Can you work these out from the model? Positions are in its coordinate system, mm. Face numbers are marked on the shaded views. A direction names the side the tool comes from. Round coordinates to 2 decimals unless told otherwise and drop trailing zeros. Write each loop counter-clockwise with the first axis right and the second up, starting at its lowest first coordinate (ties: lowest second). Pieces come first, ordered by that corner, then holes.
Q1. If we section it at C-C (x = 11): Please give me the cut outline in (y, z), plus the area to 3 significant figures.
Q2. For the marked faces 1, 2 and 3, which set-ups out of +Z, -Z, +X, -X, +Y, -Y let a thin tool reach every point of the face, with its end or its side?
Q3. If we section it at D-D (y = 6): Please give me the cut outline in (x, z), plus the area to 3 significant figures.
Q4. If we section it at B-B (z = 2.25): Please give me the cut outline in (x, y), plus the area to 3 significant figures.
Q5. I'm going to push flat-ended pins straight in: pin 1 Ø1.5 at (y, z) = (-16, 2) entering from +X; pin 2 Ø4.5 at (x, y) = (11.71, -15.62) entering from +Z; pin 3 Ø0.7 at (y, z) = (-16, 1.5) entering from -X. Where does each tip first touch, or does it pass through?
Q6. If we section it at A-A (x = 5.5): Please give me the cut outline in (y, z).
Q7. Please list where these lines run through material, in increasing order: line 1 along Y through (x, z) = (-5, 2); line 2 along X through (y, z) = (0, 2.25); line 3 along Y through (x, z) = (-6, 6.25).
from build123d import *

# Parameters (mm, degrees)
SKETCH1_R           = 16.5
SKETCH1_R_2         = 2.4
SKETCH1_R_3         = 1.4
BOSS_EXTRUDE1_DEPTH = 3
BOSS_EXTRUDE2_START = -3
SKETCH3_R           = 1.4
BOSS_EXTRUDE2_DEPTH = 3
SKETCH4_W           = 33
SKETCH4_H           = 12
SKETCH4_R           = 1.4
BOSS_EXTRUDE3_DEPTH = 5.5
SKETCH5_W           = 33
SKETCH5_H           = 9
CUT_EXTRUDE1_DEPTH  = 6.5
FILLET1_R           = 3
CHAMFER1_SIZE       = 1


with BuildPart() as part:
    # Sketch1 → Boss-Extrude1 (new body)
    # profile 1 of 5: a face of its own
    with BuildSketch(Plane.XY):
        with Locations((3.7111495, -7.618539739)):
            Circle(SKETCH1_R)
        with BuildLine():
            ThreePointArc((-4.2888505, -2.018539739), (-5.985906775, 2.078516536), (-1.8888505, 0.381460261))
            Line((-1.8888505, 0.381460261), (-1.8888505, 1.781460261))
            Line((-1.8888505, 1.781460261), (9.3111495, 1.781460261))
            Line((9.3111495, 1.781460261), (9.3111495, 0.381460261))
            ThreePointArc((9.3111495, 0.381460261), (11.7111495, 2.781460261), (14.1111495, 0.381460261))
            ThreePointArc((14.1111495, 0.381460261), (13.408205775, -1.315596014), (11.7111495, -2.018539739))
            Line((11.7111495, -2.018539739), (13.1111495, -2.018539739))
            Line((13.1111495, -2.018539739), (13.1111495, -13.218539739))
            Line((13.1111495, -13.218539739), (11.7111495, -13.218539739))
            ThreePointArc((11.7111495, -13.218539739), (13.408205775, -13.921483464), (14.1111495, -15.618539739))
            ThreePointArc((14.1111495, -15.618539739), (11.7111495, -18.018539739), (9.3111495, -15.618539739))
            Line((9.3111495, -15.618539739), (9.3111495, -17.018539739))
            Line((9.3111495, -17.018539739), (-1.8888505, -17.018539739))
            Line((-1.8888505, -17.018539739), (-1.8888505, -15.618539739))
            ThreePointArc((-1.8888505, -15.618539739), (-5.985906775, -17.315596014), (-4.2888505, -13.218539739))
            Line((-4.2888505, -13.218539739), (-5.6888505, -13.218539739))
            Line((-5.6888505, -13.218539739), (-5.6888505, -2.018539739))
            Line((-5.6888505, -2.018539739), (-4.2888505, -2.018539739))
        make_face(mode=Mode.SUBTRACT)
    # profile 2 of 5: a face of its own
    with BuildSketch(Plane.XY):
        with Locations((11.7111495, -15.618539739)):
            Circle(SKETCH1_R_2)
        with Locations((11.7111495, -15.618539739)):
            Circle(SKETCH1_R_3, mode=Mode.SUBTRACT)
    # profile 3 of 5: a face of its own
    with BuildSketch(Plane.XY):
        with Locations((-4.2888505, -15.618539739)):
            Circle(SKETCH1_R_2)
        with Locations((-4.2888505, -15.618539739)):
            Circle(SKETCH1_R_3, mode=Mode.SUBTRACT)
    # profile 4 of 5: a face of its own
    with BuildSketch(Plane.XY):
        with Locations((-4.2888505, 0.381460261)):
            Circle(SKETCH1_R_2)
        with Locations((-4.2888505, 0.381460261)):
            Circle(SKETCH1_R_3, mode=Mode.SUBTRACT)
    # profile 5 of 5: a face of its own
    with BuildSketch(Plane.XY):
        with Locations((11.7111495, 0.381460261)):
            Circle(SKETCH1_R_2)
        with Locations((11.7111495, 0.381460261)):
            Circle(SKETCH1_R_3, mode=Mode.SUBTRACT)
    extrude(amount=BOSS_EXTRUDE1_DEPTH)

    # Sketch3 → Boss-Extrude2 (add)
    with BuildSketch(Plane.XY.offset(3).offset(BOSS_EXTRUDE2_START)):
        with BuildLine():
            Line((-12.7888505, 46.381460261), (-12.7888505, -7.618539739))
            ThreePointArc((-12.7888505, -7.618539739), (3.7111495, 8.881460261), (20.2111495, -7.618539739))
            Line((20.2111495, -7.618539739), (20.2111495, 46.381460261))
            Line((20.2111495, 46.381460261), (-12.7888505, 46.381460261))
        make_face()
        with Locations((-8.2888505, 41.881460261)):
            Circle(SKETCH3_R, mode=Mode.SUBTRACT)
        with Locations((15.7111495, 41.881460261)):
            Circle(SKETCH3_R, mode=Mode.SUBTRACT)
    extrude(amount=BOSS_EXTRUDE2_DEPTH)

    # Sketch4 → Boss-Extrude3 (add)
    with BuildSketch(Plane.XY.offset(3)):
        with Locations((3.7111495, 40.381460261)):
            Rectangle(SKETCH4_W, SKETCH4_H)
        with Locations((-8.2888505, 41.881460261)):
            Circle(SKETCH4_R, mode=Mode.SUBTRACT)
        with Locations((15.7111495, 41.881460261)):
            Circle(SKETCH4_R, mode=Mode.SUBTRACT)
    extrude(amount=BOSS_EXTRUDE3_DEPTH)

    # Sketch5 → Cut-Extrude1 (cut)
    with BuildSketch(Plane(origin=(0, 0, 0), x_dir=(-1, 0, 0), z_dir=(0, 0, -1))):
        with Locations((-3.7111495, 41.881460261)):
            Rectangle(SKETCH5_W, SKETCH5_H)
    extrude(amount=-CUT_EXTRUDE1_DEPTH, mode=Mode.SUBTRACT)

    # Fillet1
    fillet1_edges = [part.edges().sort_by_distance(p)[0] for p in [
        (20.2111495, 46.381460261, 7.5),
        (-12.7888505, 46.381460261, 7.5),
        (3.7111495, 37.381460261, 0),
        (3.7111495, 34.381460261, 3),
    ]]
    fillet(fillet1_edges, radius=FILLET1_R)

    # Chamfer1
    chamfer1_edges = [part.edges().sort_by_distance(p)[0] for p in [
        (-9.6888505, 41.881460261, 6.5),
        (14.3111495, 41.881460261, 6.5),
    ]]
    chamfer(chamfer1_edges, length=CHAMFER1_SIZE)


solid = part.part
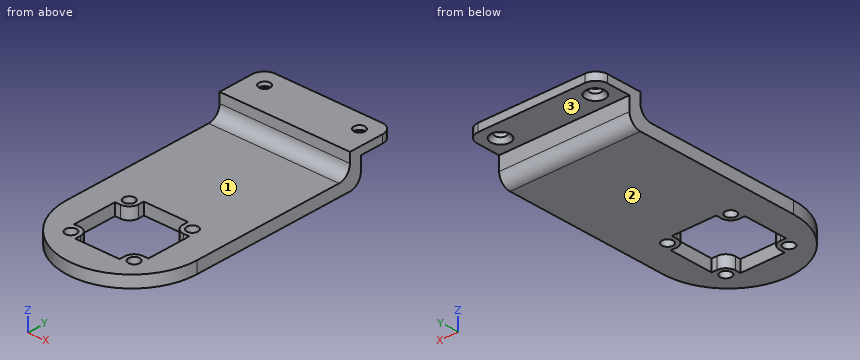
A:
1. outline: (-22.42, 0) - (-16.82, 0) - (-16.82, 3) - (-22.42, 3) - close; (-14.41, 0) - (-13.33, 0) - (-13.33, 3) - (-14.41, 3) - close; (-1.91, 0) - (-0.82, 0) - (-0.82, 3) - (-1.91, 3) - close; (1.59, 0) - (34.38, 0) arc R3 ccw to (37.38, 3) - (37.38, 6.5) - (46.38, 6.5) - (46.38, 8.5) - (34.38, 8.5) - (34.38, 6) arc R3 cw to (31.38, 3) - (1.59, 3) - close
1. area: 165 mm2
2. face 1: +Z, +X, -X, -Y
2. face 2: -Z, +X, -X, +Y, -Y
2. face 3: -Z, +X, -X, +Y
3. outline: (-12.79, 0) - (20.21, 0) - (20.21, 3) - (-12.79, 3) - close
3. area: 99.0 mm2
4. outline: (-12.79, -7.62) arc R16.5 ccw to (20.21, -7.62) - (20.21, 37.29) - (-12.79, 37.29) - close; hole circle Ø2.8 at (-4.29, -15.62); hole (-5.69, -13.22) - (-4.29, -13.22) arc R2.4 cw to (-1.89, -15.62) - (-1.89, -17.02) - (9.31, -17.02) - (9.31, -15.62) arc R2.4 cw to (11.71, -13.22) - (13.11, -13.22) - (13.11, -2.02) - (11.71, -2.02) arc R2.4 cw to (9.31, 0.38) - (9.31, 1.78) - (-1.89, 1.78) - (-1.89, 0.38) arc R2.4 cw to (-4.29, -2.02) - (-5.69, -2.02) - close; hole circle Ø2.8 at (-4.29, 0.38); hole circle Ø2.8 at (11.71, -15.62); hole circle Ø2.8 at (11.71, 0.38)
4. area: 1,580 mm2
5. pin 1: stops at x = 18.34
5. pin 2: stops at z = 3
5. pin 3: stops at x = -10.7
6. outline: (-24.02, 0) - (-17.02, 0) - (-17.02, 3) - (-24.02, 3) - close; (1.78, 0) - (34.38, 0) arc R3 ccw to (37.38, 3) - (37.38, 6.5) - (46.38, 6.5) - (46.38, 8.5) - (34.38, 8.5) - (34.38, 6) arc R3 cw to (31.38, 3) - (1.78, 3) - close
7. line 1: y = -21.63 to -16.82, -14.41 to -13.22, -2.02 to -0.82, 1.59 to 37.21
7. line 2: x = -12.79 to -5.64, -2.94 to -1.92, 9.34 to 10.36, 13.06 to 20.21
7. line 3: y = 34.38 to 37.38
